```python
from build123d import *

# Parameters (mm, degrees)
FILLET1_R                       = 1
M3X0_5_TAPPED_HOLE1_D           = 2.5
M3X0_5_TAPPED_HOLE1_CSINK_D     = 3.25
M3X0_5_TAPPED_HOLE1_CSINK_ANGLE = 90
CUT_EXTRUDE1_DEPTH              = 6


with BuildPart() as part:
    # Sketch4 → Revolve1 (revolve)
    with BuildSketch(Plane(origin=(0, 0, 0), x_dir=(0, 0, -1), z_dir=(1, 0, 0)), mode=Mode.PRIVATE) as revolve1_sk:
        Polygon((0, 16.5), (0, 17.5), (-10, 15.006719972), (-10, 8), (-5, 8), (-5, 15.253359986), align=None)
    revolve(revolve1_sk.sketch.rotate(Axis((0, 0, 0), (0, 0, 1)), 90), axis=Axis((0, 0, 0), (0, 0, 1)))

    # Fillet1
    fillet1_edges = [part.edges().sort_by_distance(p)[0] for p in [
        (15.006719972, 0, 10),
    ]]
    fillet(fillet1_edges, radius=FILLET1_R)

    # M3x0.5 Tapped Hole1 (through all)
    with Locations(Plane.XY.offset(10)):
        with Locations((8.838834765, 8.838834765), (-8.838834765, 8.838834765), (-8.838834765, -8.838834765), (8.838834765, -8.838834765)):
            CounterSinkHole(M3X0_5_TAPPED_HOLE1_D / 2, M3X0_5_TAPPED_HOLE1_CSINK_D / 2, counter_sink_angle=M3X0_5_TAPPED_HOLE1_CSINK_ANGLE)

    # Sketch9 → Cut-Extrude1 (cut)
    with BuildSketch(Plane.XY.offset(10)):
        with BuildLine():
            Line((-13.242640687, 20), (-4.621320344, 11.378679656))
            ThreePointArc((-4.621320344, 11.378679656), (-3.648050297, 10.728361402), (-2.5, 10.5))
            Line((-2.5, 10.5), (2.5, 10.5))
            ThreePointArc((2.5, 10.5), (3.648050297, 10.728361402), (4.621320344, 11.378679656))
            Line((4.621320344, 11.378679656), (13.242640687, 20))
            Line((13.242640687, 20), (-13.242640687, 20))
        make_face()
        with BuildLine():
            Line((20, 13.242640687), (11.378679656, 4.621320344))
            ThreePointArc((11.378679656, 4.621320344), (10.728361402, 3.648050297), (10.5, 2.5))
            Line((10.5, 2.5), (10.5, -2.5))
            ThreePointArc((10.5, -2.5), (10.728361402, -3.648050297), (11.378679656, -4.621320344))
            Line((11.378679656, -4.621320344), (20, -13.242640687))
            Line((20, -13.242640687), (20, 13.242640687))
        make_face()
        with BuildLine():
            Line((13.242640687, -20), (4.621320344, -11.378679656))
            ThreePointArc((4.621320344, -11.378679656), (3.648050297, -10.728361402), (2.5, -10.5))
            Line((2.5, -10.5), (-2.5, -10.5))
            ThreePointArc((-2.5, -10.5), (-3.648050297, -10.728361402), (-4.621320344, -11.378679656))
            Line((-4.621320344, -11.378679656), (-13.242640687, -20))
            Line((-13.242640687, -20), (13.242640687, -20))
        make_face()
        with BuildLine():
            Line((-20, -13.242640687), (-11.378679656, -4.621320344))
            ThreePointArc((-11.378679656, -4.621320344), (-10.728361402, -3.648050297), (-10.5, -2.5))
            Line((-10.5, -2.5), (-10.5, 2.5))
            ThreePointArc((-10.5, 2.5), (-10.728361402, 3.648050297), (-11.378679656, 4.621320344))
            Line((-11.378679656, 4.621320344), (-20, 13.242640687))
            Line((-20, 13.242640687), (-20, -13.242640687))
        make_face()
    extrude(amount=-CUT_EXTRUDE1_DEPTH, mode=Mode.SUBTRACT)


solid = part.part
```
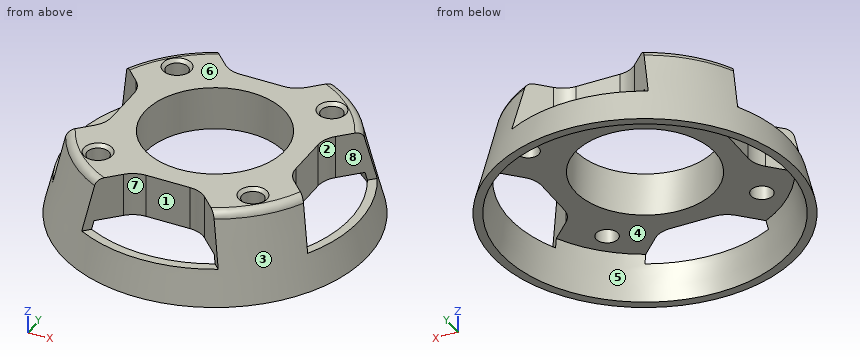
Work out the finished part from the listing and answer in its coordinate system (mm). Face numbers are marked on the shaded views. A direction names the side the tool comes from. Give positions to 0.01 mm unless a question says otherwise; leave off trailing zeros. Loops run counter-clockwise (first coordinate to the right, second up) from the corner with the lowest first, then second, coordinate; pieces in that order, holes last. Notation, with made-up numbers: (42, -21) -> (68, -21) arc R27 cw to (68, 5) -> close; hole circle Ø6 at (-27.5, 78). An arc over 180 degrees is marked (long way). Put each result on its own line as item: value. Start each with the question number.
Item 1: Each of these flat-tipped pins is pushed along its axis until it touches: P1, Ø1, axis at y = 6.5, z = 5.5, coming from the -X side; P2, Ø2, axis at x = -15, y = -3, coming from the +Z side; P3, Ø4, axis at y = 1, z = 6.5, coming from the -X side. Where does it stop, or does it pass through?
Item 2: The part is cut by section C-C (z = 2.75). Give the vertices of the cut face in (x, y), then the cut area to 3 significant figures.
Item 3: The part is cut by section A-A (x = 0). Give the vertices of the cut face in (y, z).
Item 4: Which of the six approach directions +Z, -Z, +X, -X, +Y, -Y give full straight-line access (tool end or side, diameter ignored) to the marked faces 1, 2, 3 and 4?
Item 5: The mould has two halves that part along X. Classify the marked faces 5, 6, 7 and 8: released by +X, released by -X, zero draft, split by the parting line, or undercut.
Item 6: Find the intervals of material crossed by L1, parallel to Y at x = 0, z = 8.75; L2, parallel to Y at x = 9.5, z = 7.5; L3, parallel to Z at x = -10, y = -5, in increasing order. Write a range as [from, to].
Answers below:
1. P1: x = -13.76
1. P2: z = 4
1. P3: x = -10.54
2. outline: circle Ø33.63 at (0, 0); hole circle Ø31.63 at (0, 0)
2. area: 103 mm2
3. outline: (-17.5, 0) -> (-16.5, 0) -> (-15.5, 4) -> (-16.5, 4) -> close; (-10.5, 5) -> (-8, 5) -> (-8, 10) -> (-10.5, 10) -> close; (8, 5) -> (10.5, 5) -> (10.5, 10) -> (8, 10) -> close; (15.5, 4) -> (16.5, 0) -> (17.5, 0) -> (16.5, 4) -> close
4. face 1: +Z, -Z, -Y
4. face 2: +Z, -Z, +X
4. face 3: +Z
4. face 4: -Z
5. face 5: undercut
5. face 6: zero draft
5. face 7: undercut
5. face 8: released by +X
6. L1: [-10.5, -8], [8, 10.5]
6. L2: [-12.41, -9.9], [-7.78, 7.78], [9.9, 12.41]
6. L3: [5, 10]
